```python
from build123d import *

# Parameters (mm, degrees)
SKETCH1_W           = 60
SKETCH1_H           = 90
BOSS_EXTRUDE1_DEPTH = 10
SKETCH2_R           = 30
BOSS_EXTRUDE2_DEPTH = 30


with BuildPart() as part:
    # Sketch1 → Boss-Extrude1 (new body)
    with BuildSketch(Plane.XY):
        Rectangle(SKETCH1_W, SKETCH1_H)
    extrude(amount=BOSS_EXTRUDE1_DEPTH)

    # Sketch2 → Boss-Extrude2 (add)
    with BuildSketch(Plane(origin=(0, 0, 0), x_dir=(-1, 0, 0), z_dir=(0, 0, -1))):
        Circle(SKETCH2_R)
        with BuildLine():
            Line((4, -13.912685387), (4, -13.325269778))
            ThreePointArc((4, -13.325269778), (0, 13.912685387), (-4, -13.325269778))
            Line((-4, -13.325269778), (-4, -13.912685387))
            Line((-4, -13.912685387), (-4, -16.912685387))
            Line((-4, -16.912685387), (4, -16.912685387))
            Line((4, -16.912685387), (4, -13.912685387))
        make_face(mode=Mode.SUBTRACT)
    extrude(amount=BOSS_EXTRUDE2_DEPTH)


solid = part.part
```
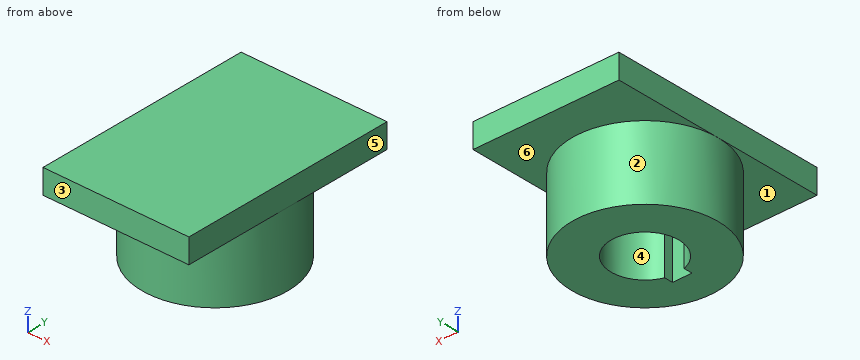
Input: part model. Units: mm. Frame: model coordinates. Face numbers are marked on the shaded views. A direction names the side the tool comes from. Give positions to 0.01 mm unless a question says otherwise; leave off trailing zeros. Order: outer loops, then holes, each group sorted by start corner. A loop starts at its lowest first (then second) coordinate and runs counter-clockwise, first axis right, second up.
1. Cut plane C-C (x = 0). Return loops of the section in (y, z), and give its area (3 significant figures).
Computed:
outline: (-45, 0) - (-30, 0) - (-30, -30) - (-16.91, -30) - (-16.91, 0) - (13.91, 0) - (13.91, -30) - (30, -30) - (30, 0) - (45, 0) - (45, 10) - (-45, 10) - close
area: 1,780 mm2
2. Pin query (flat end, axial travel): pin 1 Ø3 at (x, z) = (-10.5, -12) entering from +Y; pin 2 Ø1.8 at (y, z) = (-16, -17) entering from -X; pin 3 Ø5 at (x, z) = (14, -21) entering from -Y; pin 4 Ø2 at (y, z) = (-34, -1.5) entering from -X (3 decimals). Return the tip coordinate at first contact, or that it passes through.
Computed:
pin 1: stops at y = 28.62
pin 2: stops at x = -25.92
pin 3: stops at y = -27.71
pin 4: passes through
3. Cut plane B-B (z = -9). Return loops of the section in (x, y).
Computed:
outline: circle Ø60 at (0, 0); hole (-4, -16.91) - (4, -16.91) - (4, -13.33) arc R13.91 ccw (long way) to (-4, -13.33) - close
4. Line query: probe 1 along Z at (x, y) = (7, -6.5); probe 2 along X at (y, z) = (-9, -3); probe 3 along Y at (x, z) = (-7, -10.5). Output: solid intervals per line, ascending.
Computed:
probe 1: z = 0 to 10
probe 2: x = -28.62 to -10.61, 10.61 to 28.62
probe 3: y = -29.17 to -12.02, 12.02 to 29.17
5. Cut plane D-D (y = 33.5). Return loops of the section in (x, z).
Computed:
outline: (-30, 0) - (30, 0) - (30, 10) - (-30, 10) - close
6. Draft query along X for the marked faces 4, 5 and 6. Return one class per face: released by +X, released by -X, zero draft, split by the parting line, or undercut.
Computed:
face 4: undercut
face 5: released by +X
face 6: zero draft
7. Cut plane A-A (x = -18). Return loops of the section in (y, z), and give its area (3 significant figures).
Computed:
outline: (-45, 0) - (-24, 0) - (-24, -30) - (24, -30) - (24, 0) - (45, 0) - (45, 10) - (-45, 10) - close
area: 2,340 mm2
8. Set-up query: the marked faces 1, 2 and 3. Return all of +Z, -Z, +X, -X, +Y, -Y with unobstructed straight access to the full face (end or side cutting, diameter ignored); none if empty.
Computed:
face 1: -Z, -Y
face 2: -Z
face 3: +Z, -Z, +X, -X, -Y
